Can you work these out from the drawing? Everything is in mm from the part's minimum corner. A direction names the side the tool comes from. Round coordinates to 2 decimals unless told otherwise and drop trailing zeros. Loops run counter-clockwise (first coordinate to the right, second up) from the corner with the lowest first, then second, coordinate; pieces in that order, holes last. Notation, with made-up numbers: (-33.5, 58) -> (-11.5, 58) arc R11 cw to (-11.5, 70) -> close; hole circle Ø9 at (62, 1.25). An arc over 180 degrees is marked (long way). One line per item, written item: value.
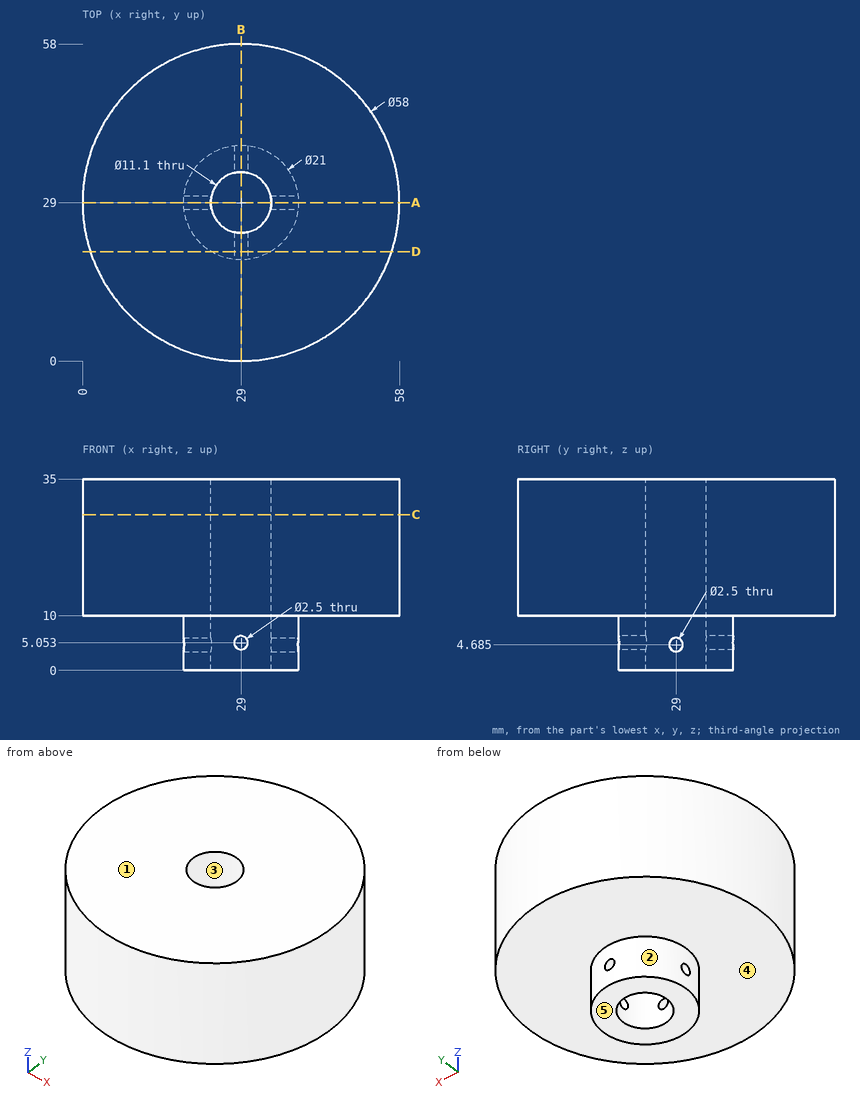
Item 1: Will these pins go through, and if not, where does the flat tip stop? pin 1 Ø4 at (x, z) = (29, 5.05) entering from +Y; pin 2 Ø2 at (y, z) = (7, 25.5) entering from -X; pin 3 Ø10 at (y, z) = (46.5, 17.5) entering from +X.
Output:
pin 1: stops at y = 39.5
pin 2: stops at x = 9
pin 3: stops at x = 55.17
Item 2: If we section it at C-C on z = 28.5: List the corners of the cut face in (x, y) for me.
Output:
outline: circle Ø58 at (29, 29); hole circle Ø11.1 at (29, 29)
Item 3: If we mould it in two halves opening along Y, with no side actions, what happens to the marked faces 1, 2 and 3? For each: released by +Y, released by -Y, zero draft, split by the parting line, or undercut.
Output:
face 1: zero draft
face 2: split by the parting line
face 3: undercut
Item 4: If we section it at A-A on y = 29: Count the separate pieces of the cut face and the enclosed holes in it, plus the area to 3 significant figures.
Output:
separate pieces: 4
enclosed holes: 0
area: 1,250 mm²
Item 5: I need wall thicknesses on line 1 (Z direction, x = 29, y = 19.65); line 2 (Z direction, x = 33.5, y = 12.5); line 3 (X direction, y = 33, z = 9). Which ranges of each line are inside material? Lowest first, please. Write a range as from..to.
Output:
line 1: z = 0..3.8, 6.3..35
line 2: z = 10..35
line 3: x = 19.29..25.15, 32.85..38.71
Item 6: If we section it at D-D on y = 20: List the corners of the cut face in (x, z) for me, plus the area to 3 significant figures.
Output:
outline: (1.43, 10) -> (23.59, 10) -> (23.59, 0) -> (34.41, 0) -> (34.41, 10) -> (56.57, 10) -> (56.57, 35) -> (1.43, 35) -> close; hole circle Ø2.5 at (29, 5.05)
area: 1,480 mm²
Item 7: If we section it at B-B on x = 29: List the corners of the cut face in (y, z) for me, plus the area to 3 significant figures.
Output:
outline: (0, 10) -> (18.5, 10) -> (18.5, 6.3) -> (23.45, 6.3) -> (23.45, 35) -> (0, 35) -> close; (18.5, 0) -> (23.45, 0) -> (23.45, 3.8) -> (18.5, 3.8) -> close; (34.55, 0) -> (39.5, 0) -> (39.5, 3.8) -> (34.55, 3.8) -> close; (34.55, 6.3) -> (39.5, 6.3) -> (39.5, 10) -> (58, 10) -> (58, 35) -> (34.55, 35) -> close
area: 1,250 mm²
Item 8: For the marked faces 4 and 5, which set-ups out of +Z, -Z, +X, -X, +Y, -Y let a thin tool reach every point of the face, with its end or its side?
Output:
face 4: -Z
face 5: -Z, +X, -X, +Y, -Y
